Check sheet for the modelled part. Datum: model origin and axes. Units: mm. Give positions to 0.01 mm unless a question says otherwise; leave off trailing zeros. Write each loop counter-clockwise with the first axis right and the second up, starting at its lowest first coordinate (ties: lowest second). Pieces come first, ordered by that corner, then holes. Notation, with made-up numbers: M 0,30.25 L 37,30.25 A20 cw 37,43.25 Z; hole C 22,-15 d4. An arc over 180 degrees is marked long. Use CSV: the item, a comma, the result in double quotes. Start each with the question number.
1. Cross-section at C-C, the plane z = 13.5. Enter the section's corners in (x, y).
2. Cross-section at D-D, the plane z = 3.5. Enter the section's corners in (x, y), and give its area (3 significant figures).
3. Cross-section at A-A, the plane x = 0. Enter the section's corners in (y, z).
4. Cross-section at B-B, the plane y = 1.2. Enter the section's corners in (x, z).
5. Scan lines: line 1 (X direction, y = 1.3, z = -13.5); line 2 (X direction, y = 1.35, z = 0); line 3 (Z direction, x = -14, y = 1.65). Record each from-to range of solid material in increasing order.
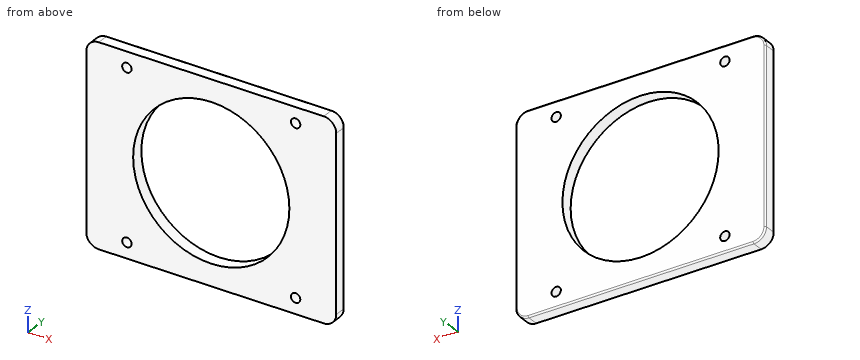
from build123d import *

# Parameters (mm, degrees)
SKETCH1_W           = 40
SKETCH1_H           = 32
SKETCH1_R           = 12.5
SKETCH1_R_2         = 0.75
BOSS_EXTRUDE1_DEPTH = 2
FILLET1_R           = 0.25
FILLET2_R           = 2


with BuildPart() as part:
    # Sketch1 → Boss-Extrude1 (new body)
    with BuildSketch(Plane(origin=(0, 0, 0), x_dir=(1, 0, 0), z_dir=(0, 1, 0))):
        Rectangle(SKETCH1_W, SKETCH1_H)
        with Locations(Location((0, 0, 0), (0, 0, 270))):
            Circle(SKETCH1_R, mode=Mode.SUBTRACT)
        with Locations(Location((-13.5, 13.5, 0), (0, 0, 270))):
            Circle(SKETCH1_R_2, mode=Mode.SUBTRACT)
        with Locations(Location((13.5, 13.5, 0), (0, 0, 270))):
            Circle(SKETCH1_R_2, mode=Mode.SUBTRACT)
        with Locations(Location((13.5, -13.5, 0), (0, 0, 270))):
            Circle(SKETCH1_R_2, mode=Mode.SUBTRACT)
        with Locations(Location((-13.5, -13.5, 0), (0, 0, 270))):
            Circle(SKETCH1_R_2, mode=Mode.SUBTRACT)
    extrude(amount=BOSS_EXTRUDE1_DEPTH)

    # Fillet1
    fillet1_edges = [part.edges().sort_by_distance(p)[0] for p in [
        (-20, 2, 0),
        (0, 2, 16),
        (20, 2, 0),
        (0, 2, -16),
    ]]
    fillet(fillet1_edges, radius=FILLET1_R)

    # Fillet2
    # the kernel refuses this fillet: 2 mm, written as the material it takes off along each edge
    with BuildSketch(Plane(origin=(-18, 2, 14), x_dir=(-1, 0, 0), z_dir=(0, 0, -1))) as fillet2_piece_1:
        with BuildLine():
            CenterArc((1.75, -0.25), 0.25, 0, 90)
            Line((2, -0.25), (2, 0))
            Line((2, 0), (1.75, 0))
        make_face()
    revolve(axis=Axis((-18, 2, 14), (0, 1, 0)), revolution_arc=90, mode=Mode.SUBTRACT)
    with BuildSketch(Plane(origin=(-18, 2, -14), x_dir=(0, 0, -1), z_dir=(1, 0, 0))) as fillet2_piece_2:
        with BuildLine():
            CenterArc((1.75, -0.25), 0.25, 0, 90)
            Line((2, -0.25), (2, 0))
            Line((2, 0), (1.75, 0))
        make_face()
    revolve(axis=Axis((-18, 2, -14), (0, 1, 0)), revolution_arc=90, mode=Mode.SUBTRACT)
    with BuildSketch(Plane(origin=(18, 2, 14), x_dir=(0, 0, 1), z_dir=(-1, 0, 0))) as fillet2_piece_3:
        with BuildLine():
            CenterArc((1.75, -0.25), 0.25, 0, 90)
            Line((2, -0.25), (2, 0))
            Line((2, 0), (1.75, 0))
        make_face()
    revolve(axis=Axis((18, 2, 14), (0, 1, 0)), revolution_arc=90, mode=Mode.SUBTRACT)
    with BuildSketch(Plane(origin=(18, 2, -14), x_dir=(1, 0, 0), z_dir=(0, 0, 1))) as fillet2_piece_4:
        with BuildLine():
            CenterArc((1.75, -0.25), 0.25, 0, 90)
            Line((2, -0.25), (2, 0))
            Line((2, 0), (1.75, 0))
        make_face()
    revolve(axis=Axis((18, 2, -14), (0, 1, 0)), revolution_arc=90, mode=Mode.SUBTRACT)
    with BuildSketch(Plane(origin=(20, -5, -16), x_dir=(0, 0, 1), z_dir=(0, 1, 0)), Plane(origin=(20, -5, 16), x_dir=(-1, 0, 0), z_dir=(0, 1, 0))) as fillet2_piece_5:
        with BuildLine():
            CenterArc((FILLET2_R, -FILLET2_R), FILLET2_R, 90, 90)
            Line((0, -FILLET2_R), (0, 0))
            Line((0, 0), (FILLET2_R, 0))
        make_face()
    extrude(amount=7, mode=Mode.SUBTRACT)
    with BuildSketch(Plane(origin=(-20, -5, -16), x_dir=(0, 0, 1), z_dir=(0, 1, 0)), Plane(origin=(-20, -5, 16), x_dir=(1, 0, 0), z_dir=(0, 1, 0))) as fillet2_piece_6:
        with BuildLine():
            CenterArc((FILLET2_R, FILLET2_R), FILLET2_R, 180, 90)
            Line((0, FILLET2_R), (0, 0))
            Line((0, 0), (FILLET2_R, 0))
        make_face()
    extrude(amount=7, mode=Mode.SUBTRACT)


solid = part.part
Worked answers:
1,outline,"M -20,0 L -14.25,0 L -14.25,2 L -19.75,2 A0.25 ccw -20,1.75 Z; M -12.75,0 L 12.75,0 L 12.75,2 L -12.75,2 Z; M 14.25,0 L 20,0 L 20,1.75 A0.25 ccw 19.75,2 L 14.25,2 Z"
2,outline,"M -20,0 L -12,0 L -12,2 L -19.75,2 A0.25 ccw -20,1.75 Z; M 12,0 L 20,0 L 20,1.75 A0.25 ccw 19.75,2 L 12,2 Z"
2,area,"32.0 mm^2"
3,outline,"M 0,-16 L 1.75,-16 A0.25 ccw 2,-15.75 L 2,-12.5 L 0,-12.5 Z; M 0,12.5 L 2,12.5 L 2,15.75 A0.25 ccw 1.75,16 L 0,16 Z"
4,outline,"M -20,-14 A2 ccw -18,-16 L 18,-16 A2 ccw 20,-14 L 20,14 A2 ccw 18,16 L -18,16 A2 ccw -20,14 Z; hole C -13.5,-13.5 d1.5; hole C -13.5,13.5 d1.5; hole C 0,0 d25; hole C 13.5,-13.5 d1.5; hole C 13.5,13.5 d1.5"
5,line 1,"x = -20 to -14.25, -12.75 to 12.75, 14.25 to 20"
5,line 2,"x = -20 to -12.5, 12.5 to 20"
5,line 3,"z = -16 to -14.06, -12.94 to 12.94, 14.06 to 16"
